Source: CAD feature listing. Evaluate the final solid. Frame: model axes, mm. A direction names the side the tool comes from. Give positions to 0.01 mm unless a question says otherwise; leave off trailing zeros. Loops run counter-clockwise (first coordinate to the right, second up) from the corner with the lowest first, then second, coordinate; pieces in that order, holes last. Notation, with made-up numbers: (89, 61) -> (126, 61) arc R12 cw to (126, 72) -> close; hole circle Ø1 at (-6.5, 56). An arc over 180 degrees is marked (long way). Return JSON: item names as keys, results as strings. Group by question number.
(1) Cut plane A-A on y = 113. Return loops of the section in (x, z), then the cut area to 3 significant figures.
(2) Access query for faces 1 (the face through (-46.78, 116.89, 3.13)), 2 (the face through (-36, 203, 0)). Directions: +Z, -Z, +X, -X, +Y, -Y. A direction counts if a zero-diameter tool reaches every point of the face in a straight line with its end or side. Return the directions, or none.
(3) Ray query, line 1 (Y direction, x = -10, z = 2); line 2 (Y direction, x = -92.5, z = 2.5); line 3 (X direction, y = 54, z = 3.5). Return the intervals inside material, ascending. Write a range as from..to.
(4) Pin query (flat end, axial travel): pin 1 (1.9 mm diameter, centred on x = -58, z = 3.5, fed in from -Y). Return the tip coordinate at first contact, or that it passes through.
(5) Cut plane B-B on z = 4. Give the number of separate pieces and of enclosed holes in the cut face, then the cut area to 3 significant figures.
(6) Draft query along X for faces 3 (the face through (-45.77, 36.21, 3.13)), 4 (the face through (-45.77, 188.61, 3.13)), 5 (the face through (-36, 203, 6.35)). Return one class per face: released by +X, released by -X, zero draft, split by the parting line, or undercut.
```python
from build123d import *

# Parameters (mm, degrees)
BOSS_EXTRUDE1_DEPTH = 6.35


with BuildPart() as part:
    # Model → Boss-Extrude1 (new body)
    with BuildSketch(Plane.XY):
        Polygon((-95.25, 386.08), (-6.35, 386.08), (-6.35, 436.88), (0, 436.88), (0, 0), (-101.6, 0), (-101.6, 436.88), (-95.25, 436.88), align=None)
        with BuildLine():
            Line((-80.76878597, 311.15), (-12.7, 311.15))
            ThreePointArc((-12.7, 311.15), (-8.209871939, 313.009871939), (-6.35, 317.5))
            Line((-6.35, 317.5), (-6.35, 363.45223644))
            ThreePointArc((-6.35, 363.45223644), (-7.711169032, 365.702115893), (-10.335793346, 365.540604607))
            Line((-10.335793346, 365.540604607), (-82.214579316, 315.778368167))
            ThreePointArc((-82.214579316, 315.778368167), (-83.193250358, 312.932654354), (-80.76878597, 311.15))
        make_face(mode=Mode.SUBTRACT)
        with BuildLine():
            Line((-95.25, 287.25223644), (-95.25, 241.3))
            ThreePointArc((-95.25, 241.3), (-93.390128061, 236.809871939), (-88.9, 234.95))
            Line((-88.9, 234.95), (-20.83121403, 234.95))
            ThreePointArc((-20.83121403, 234.95), (-18.406749642, 236.732654354), (-19.385420684, 239.578368167))
            Line((-19.385420684, 239.578368167), (-91.264206654, 289.340604607))
            ThreePointArc((-91.264206654, 289.340604607), (-93.888830968, 289.502115893), (-95.25, 287.25223644))
        make_face(mode=Mode.SUBTRACT)
        with BuildLine():
            Line((-80.76878597, 158.75), (-12.7, 158.75))
            ThreePointArc((-12.7, 158.75), (-8.209871939, 160.609871939), (-6.35, 165.1))
            Line((-6.35, 165.1), (-6.35, 211.05223644))
            ThreePointArc((-6.35, 211.05223644), (-7.711169032, 213.302115893), (-10.335793346, 213.140604607))
            Line((-10.335793346, 213.140604607), (-82.214579316, 163.378368167))
            ThreePointArc((-82.214579316, 163.378368167), (-83.193250358, 160.532654354), (-80.76878597, 158.75))
        make_face(mode=Mode.SUBTRACT)
        with BuildLine():
            Line((-20.83121403, 222.25), (-88.9, 222.25))
            ThreePointArc((-88.9, 222.25), (-93.390128061, 220.390128061), (-95.25, 215.9))
            Line((-95.25, 215.9), (-95.25, 169.94776356))
            ThreePointArc((-95.25, 169.94776356), (-93.888830968, 167.697884107), (-91.264206654, 167.859395393))
            Line((-91.264206654, 167.859395393), (-19.385420684, 217.621631833))
            ThreePointArc((-19.385420684, 217.621631833), (-18.406749642, 220.467345646), (-20.83121403, 222.25))
        make_face(mode=Mode.SUBTRACT)
        with BuildLine():
            Line((-82.214579316, 293.821631833), (-10.335793346, 244.059395393))
            ThreePointArc((-10.335793346, 244.059395393), (-7.711169032, 243.897884107), (-6.35, 246.14776356))
            Line((-6.35, 246.14776356), (-6.35, 292.1))
            ThreePointArc((-6.35, 292.1), (-8.209871939, 296.590128061), (-12.7, 298.45))
            Line((-12.7, 298.45), (-80.76878597, 298.45))
            ThreePointArc((-80.76878597, 298.45), (-83.193250358, 296.667345646), (-82.214579316, 293.821631833))
        make_face(mode=Mode.SUBTRACT)
        with BuildLine():
            Line((-95.25, 134.85223644), (-95.25, 88.9))
            ThreePointArc((-95.25, 88.9), (-93.390128061, 84.409871939), (-88.9, 82.55))
            Line((-88.9, 82.55), (-20.83121403, 82.55))
            ThreePointArc((-20.83121403, 82.55), (-18.406749642, 84.332654354), (-19.385420684, 87.178368167))
            Line((-19.385420684, 87.178368167), (-91.264206654, 136.940604607))
            ThreePointArc((-91.264206654, 136.940604607), (-93.888830968, 137.102115893), (-95.25, 134.85223644))
        make_face(mode=Mode.SUBTRACT)
        with BuildLine():
            Line((-80.76878597, 6.35), (-12.7, 6.35))
            ThreePointArc((-12.7, 6.35), (-8.209871939, 8.209871939), (-6.35, 12.7))
            Line((-6.35, 12.7), (-6.35, 58.65223644))
            ThreePointArc((-6.35, 58.65223644), (-7.711169032, 60.902115893), (-10.335793346, 60.740604607))
            Line((-10.335793346, 60.740604607), (-82.214579316, 10.978368167))
            ThreePointArc((-82.214579316, 10.978368167), (-83.193250358, 8.132654354), (-80.76878597, 6.35))
        make_face(mode=Mode.SUBTRACT)
        with BuildLine():
            Line((-20.83121403, 69.85), (-88.9, 69.85))
            ThreePointArc((-88.9, 69.85), (-93.390128061, 67.990128061), (-95.25, 63.5))
            Line((-95.25, 63.5), (-95.25, 17.54776356))
            ThreePointArc((-95.25, 17.54776356), (-93.888830968, 15.297884107), (-91.264206654, 15.459395393))
            Line((-91.264206654, 15.459395393), (-19.385420684, 65.221631833))
            ThreePointArc((-19.385420684, 65.221631833), (-18.406749642, 68.067345646), (-20.83121403, 69.85))
        make_face(mode=Mode.SUBTRACT)
        with BuildLine():
            Line((-20.83121403, 374.65), (-88.9, 374.65))
            ThreePointArc((-88.9, 374.65), (-93.390128061, 372.790128061), (-95.25, 368.3))
            Line((-95.25, 368.3), (-95.25, 322.34776356))
            ThreePointArc((-95.25, 322.34776356), (-93.888830968, 320.097884107), (-91.264206654, 320.259395393))
            Line((-91.264206654, 320.259395393), (-19.385420684, 370.021631833))
            ThreePointArc((-19.385420684, 370.021631833), (-18.406749642, 372.867345646), (-20.83121403, 374.65))
        make_face(mode=Mode.SUBTRACT)
        with BuildLine():
            Line((-82.214579316, 141.421631833), (-10.335793346, 91.659395393))
            ThreePointArc((-10.335793346, 91.659395393), (-7.711169032, 91.497884107), (-6.35, 93.74776356))
            Line((-6.35, 93.74776356), (-6.35, 139.7))
            ThreePointArc((-6.35, 139.7), (-8.209871939, 144.190128061), (-12.7, 146.05))
            Line((-12.7, 146.05), (-80.76878597, 146.05))
            ThreePointArc((-80.76878597, 146.05), (-83.193250358, 144.267345646), (-82.214579316, 141.421631833))
        make_face(mode=Mode.SUBTRACT)
    extrude(amount=BOSS_EXTRUDE1_DEPTH)


solid = part.part
```
Answers:
{
 "1": {"outline": "(-101.6, 0) -> (-95.25, 0) -> (-95.25, 6.35) -> (-101.6, 6.35) -> close; (-56.68, 0) -> (-41.16, 0) -> (-41.16, 6.35) -> (-56.68, 6.35) -> close; (-6.35, 0) -> (0, 0) -> (0, 6.35) -> (-6.35, 6.35) -> close", "area": "179 mm²"},
 "2": {"face 1": "+Z, -Z", "face 2": "-Z, +X, -X, +Y, -Y"},
 "3": {"line 1": "0..6.95, 60.94..91.46, 145.45..159.35, 213.34..243.86, 297.85..311.75, 365.74..386.08", "line 2": "0..15.02, 68.73..83.67, 137.38..167.42, 221.13..236.07, 289.78..319.82, 373.53..386.08", "line 3": "-101.6..-95.25, -35.59..-20.07, -6.35..0"},
 "4": {"pin 1": "y = 0"},
 "5": {"separate pieces": "1", "enclosed holes": "10", "area": "16,500 mm²"},
 "6": {"face 3": "undercut", "face 4": "undercut", "face 5": "zero draft"}
}
